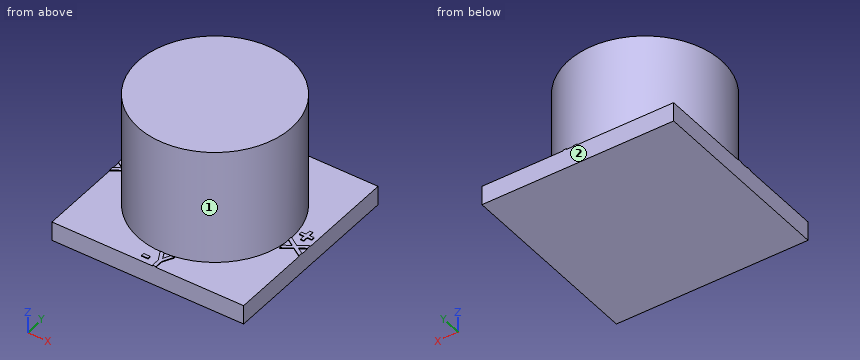
```python
from build123d import *

# Parameters (mm, degrees)
SKETCH3_R           = 200
BOSS_EXTRUDE3_DEPTH = 300
BOSS_EXTRUDE4_START = -300
SKETCH3_3_W         = 500
SKETCH3_3_H         = 500
BOSS_EXTRUDE4_DEPTH = 50
SKETCH4_W           = 8.166666666
SKETCH4_H           = 16.961538461
SKETCH4_W_2         = 16.961538462
SKETCH4_H_2         = 8.166666666
BOSS_EXTRUDE5_DEPTH = 2


with BuildPart() as part:
    # Sketch3 → Boss-Extrude3 (new body)
    with BuildSketch(Plane.XY):
        Circle(SKETCH3_R)
    extrude(amount=-BOSS_EXTRUDE3_DEPTH)

    # Sketch3<3> → Boss-Extrude4 (add)
    with BuildSketch(Plane.XY.offset(BOSS_EXTRUDE4_START)):
        Rectangle(SKETCH3_3_W, SKETCH3_3_H)
    extrude(amount=-BOSS_EXTRUDE4_DEPTH)

    # Sketch4 → Boss-Extrude5 (add)
    with BuildSketch(Plane.XY.offset(-300)):
        Polygon((228.205128205, 25.641025641), (240.384615385, 25.641025641), (240.384615385, 17.307692308), (228.205128205, 17.307692308), (228.205128205, 4.487179487), (219.871794872, 4.487179487), (219.871794872, 17.307692308), (207.692307692, 17.307692308), (207.692307692, 25.641025641), (219.871794872, 25.641025641), (219.871794872, 38.461538462), (228.205128205, 38.461538462), align=None)
        Polygon((250, -2.073317308), (250, -12.650240385), (233.944310897, -23.096955128), (250, -33.563701923), (250, -44.150641026), (225.821314103, -28.385416667), (200, -45.192307692), (200, -34.615384615), (217.708333333, -23.096955128), (200, -11.548477564), (200, -0.961538462), (225.831330128, -17.80849359), align=None)
        Polygon((-25.320512821, 228.205128205), (-25.320512821, 240.384615385), (-16.987179487, 240.384615385), (-16.987179487, 228.205128205), (-4.166666667, 228.205128205), (-4.166666667, 219.871794872), (-16.987179487, 219.871794872), (-16.987179487, 207.692307692), (-25.320512821, 207.692307692), (-25.320512821, 219.871794872), (-38.141025641, 219.871794872), (-38.141025641, 228.205128205), align=None)
        Polygon((1.282051282, 250), (11.268028846, 250), (20.192307692, 232.461939103), (29.116586538, 250), (39.102564103, 250), (24.679487179, 221.654647436), (24.679487179, 200), (15.705128205, 200), (15.705128205, 221.654647436), align=None)
        Polygon((-201, 6.763020833), (-201, -3.602363782), (-216.734575321, -13.840144231), (-201, -24.09755609), (-201, -34.47275641), (-224.695112179, -19.022836538), (-250, -35.493589744), (-250, -25.128205128), (-232.645833333, -13.840144231), (-250, -2.522636218), (-250, 7.852564103), (-224.685296474, -8.657451923), align=None)
        with Locations((-232.096153846, 23.557692308)):
            Rectangle(SKETCH4_W, SKETCH4_H)
        with Locations((-17.58974359, -232.096153846)):
            Rectangle(SKETCH4_W_2, SKETCH4_H_2)
        Polygon((-1.884615385, -201), (7.901642628, -201), (16.647435897, -218.187299679), (25.393229167, -201), (35.179487179, -201), (21.044871795, -228.778445513), (21.044871795, -250), (12.25, -250), (12.25, -228.778445513), align=None)
    extrude(amount=BOSS_EXTRUDE5_DEPTH)


solid = part.part
```
The model under review builds one solid part; all positions refer to its coordinate system, in mm. Face numbers are marked on the shaded views. A direction names the side the tool comes from. Round coordinates to 2 decimals unless told otherwise and drop trailing zeros. Order: outer loops, then holes, each group sorted by start corner. A loop starts at its lowest first (then second) coordinate and runs counter-clockwise, first axis right, second up.
Item 1: To check wall thickness, follow probe 1 along Z at (x, y) = (-196, 229.5); probe 2 along Y at (x, z) = (2.5, -83); probe 3 along Z at (x, y) = (-22, 227). State the ranges of each line that lie inside material, in increasing order.
Working result:
probe 1: z = -350 to -300
probe 2: y = -199.98 to 199.98
probe 3: z = -350 to -298
Item 2: For pin 1 (0.6 mm diameter, centred on x = -12.5, z = -299, fed in from +Y); pin 2 (10 mm diameter, centred on y = -141, z = -50.5, fed in from +X); pin 3 (2 mm diameter, centred on y = 35, z = -298.5, fed in from +X), all flat-tipped, find the tip position at first contact; note any pin that passes through.
Working result:
pin 1: stops at y = 228.21
pin 2: stops at x = 146.64
pin 3: stops at x = 228.21
Item 3: Add section A-A, the plane y = 67. State the section outline as (x, z) points, and give its area (3 significant figures).
Working result:
outline: (-250, -350) - (250, -350) - (250, -300) - (188.44, -300) - (188.44, 0) - (-188.44, 0) - (-188.44, -300) - (-250, -300) - close
area: 138,000 mm2
Item 4: Machinability: for the marked faces 1 and 2, which of the approach directions +Z, -Z, +X, -X, +Y, -Y give a long, thin tool a straight path to every point of the face, cutting with its end or side? Answer none if there is none.
Working result:
face 1: +Z
face 2: +Z, -Z, +X, -X, +Y
Item 5: Add section C-C, the plane z = -59.5. State the section outline as (x, y) points, and give its area (3 significant figures).
Working result:
outline: circle Ø400 at (0, 0)
area: 126,000 mm2
Item 6: Add section B-B, the plane x = -99. State the section outline as (y, z) points, and give its area (3 significant figures).
Working result:
outline: (-250, -350) - (250, -350) - (250, -300) - (173.78, -300) - (173.78, 0) - (-173.78, 0) - (-173.78, -300) - (-250, -300) - close
area: 129,000 mm2
